Geometry check sheet. Reference: the model listing, model coordinates, mm. Coordinates: 2 decimals unless noted, no trailing zeros. Write each loop counter-clockwise with the first axis right and the second up, starting at its lowest first coordinate (ties: lowest second). Pieces come first, ordered by that corner, then holes. Notation, with made-up numbers: (82.5, 19.5) -> (115.5, 19.5) arc R6 ccw to (115.5, 25.5) -> close; hole circle Ø6 at (40, 12). An arc over 180 degrees is marked (long way). One line per question, with ' | ' between items.
from build123d import *

# Parameters (mm, degrees)
SKETCH_1_R      = 16.1
SKETCH_1_R_2    = 15.1
EXTRUDE_1_DEPTH = 2.5
SKETCH_3_R      = 1
FILLET_1_R      = 1


with BuildPart() as part:
    # 草图1 → 凸台-拉伸1 (new body, symmetric)
    with BuildSketch(Plane.XY):
        Circle(SKETCH_1_R)
        Circle(SKETCH_1_R_2, mode=Mode.SUBTRACT)
    extrude(amount=EXTRUDE_1_DEPTH, both=True)

    # 草图3 → 切除-旋转1 (revolve, cut)
    with BuildSketch(Plane(origin=(0, 0, 0), x_dir=(1, 0, 0), z_dir=(0, 1, 0))):
        with Locations((-14.6, 0)):
            Circle(SKETCH_3_R)
    revolve(axis=Axis((0, 0, 2.5), (0, 0, -1)), mode=Mode.SUBTRACT)

    # 圆角1
    fillet_1_edges = [part.edges().sort_by_distance(p)[0] for p in [
        (0, 15.1, 0.866025404),
        (0, -15.1, -0.866025404),
    ]]
    fillet(fillet_1_edges, radius=FILLET_1_R)


solid = part.part
1. Material ranges on line 1 (Y direction, x = 0, z = -2.1); line 2 (Y direction, x = -12.5, z = -0.6) (3 decimals); line 3 (X direction, y = -7, z = -0.2), recorded low to high. Write a range as from..to.
Worked answers:
line 1: -16.1..-15.1, 15.1..16.1 | line 2: -10.147..-8.995, 8.995..10.147 | line 3: -14.5..-13.92, 13.92..14.5
2. Go/stop test with flat-tipped pins: P1, Ø1.5, axis at x = -10, z = -1, coming from the +Y side; P2, Ø1, axis at y = -2.5, z = -0.5, coming from the -X side; P3, Ø1.5, axis at x = -5, z = 0.5, coming from the +Y side. Record where each tip stops, or that it passes through.
Worked answers:
P1: y = 13.18 | P2: x = -15.98 | P3: y = 15.53
3. Cross-section at A-A on z = 1.7. Record the boundary of the cut face in (x, y).
Worked answers:
outline: circle Ø32.2 at (0, 0); hole circle Ø30.2 at (0, 0)
4. Mould release check, pull along Y, two halves, no side actions. Record for faces 1 (the face through (-3.27, -14.74, -1.92)), 2 (the face through (-3.27, -14.74, 1.9)), 3 (the face through (15.357, 4.836, 0.035)): released by +Y, released by -Y, zero draft, split by the parting line, or undercut.
Worked answers:
face 1: undercut | face 2: undercut | face 3: split by the parting line
5. Cross-section at B-B on z = -0.15. Record the boundary of the cut face in (x, y).
Worked answers:
outline: circle Ø32.2 at (0, 0); hole circle Ø31.18 at (0, 0)
